Geometry check sheet. Reference: the model listing, model coordinates, mm. A direction names the side the tool comes from. Round coordinates to 2 decimals unless told otherwise and drop trailing zeros. Write each loop counter-clockwise with the first axis right and the second up, starting at its lowest first coordinate (ties: lowest second). Pieces come first, ordered by that corner, then holes. Notation, with made-up numbers: M 8.25,45 L 13.25,45 A30 ccw 13.25,77 Z; hole C -31.5,28.5 d5. An arc over 180 degrees is marked long. Answer in a Markdown table with one row per item. Add a question column.
from build123d import *

# Parameters (mm, degrees)
F0_W     = 96.5
F0_H     = 77
F1_DEPTH = 1.6
F2_W     = 81
F2_H     = 67
F3_DEPTH = 3.3
F4_W     = 45
F4_H     = 49
F5_DEPTH = 6.5


with BuildPart() as f1:
    # F0 (on Right) → F1 (new body, symmetric)
    with BuildSketch(Plane.YZ):
        Rectangle(F0_W, F0_H)
    extrude(amount=F1_DEPTH, both=True)

    # F2 (on face) → F3 (join)
    with BuildSketch(Plane.YZ.offset(1.6)):
        with Locations((-4.75, -5)):
            Rectangle(F2_W, F2_H)
    extrude(amount=F3_DEPTH)

    # F4 (on face) → F5 (join)
    with BuildSketch(Plane.YZ.offset(4.9)):
        with Locations((-22.75, -14)):
            Rectangle(F4_W, F4_H)
    extrude(amount=F5_DEPTH)


solid = f1.part
Item 1: Section check A-A, the plane z = 27. Record the boundary of the cut face in (x, y).
Item 2: Gauge pin test, flat ends, axial feed: pin 1 Ø1.6 at (x, y) = (4, -25) entering from +Z; pin 2 Ø5 at (x, y) = (9, -28.5) entering from +Z; pin 3 Ø1 at (x, z) = (8.5, 3) entering from +Y. Record the tip position at first contact, or that the pin passes through.
Item 3: Access from +Z, -Z, +X, -X, +Y, -Y to the whole of each face (thin tool, end or side, straight path). Record for faces 1 (the flat face through (0, 48.25, -1)), 2 (the flat face through (6, -45.25, -13)), 3 (the flat face through (3, 35.75, -5)), 4 (the flat face through (3, -5, 28.5)), 5 (the flat face through (0, -48.25, -1)).
Item 4: Scan lines: probe 1 along Z at (x, y) = (3.5, 30.5); probe 2 along Y at (x, z) = (10.25, 8); probe 3 along X at (y, z) = (-21, 17). Record each from-to range of solid material in increasing order. Write a range as from..to.
Item 5: Section check C-C, the plane x = 9.5. Record the boundary of the cut face in (y, z), and give its area (4 significant figures).
Item 6: Section check B-B, the plane y = -15. Record the boundary of the cut face in (x, z), and give its area (3 significant figures).
Item 7: Section check D-D, the plane y = 30. Record the boundary of the cut face in (x, z).
Result sheet:
| question | item | result |
|---|---|---|
| 1 | outline | M -1.6,-48.25 L 1.6,-48.25 L 1.6,-45.25 L 4.9,-45.25 L 4.9,35.75 L 1.6,35.75 L 1.6,48.25 L -1.6,48.25 Z |
| 2 | pin 1 | stops at z = 28.5 |
| 2 | pin 2 | stops at z = 10.5 |
| 2 | pin 3 | stops at y = -0.25 |
| 3 | face 1 | +Z, -Z, +X, -X, +Y |
| 3 | face 2 | +Z, -Z, +X, -Y |
| 3 | face 3 | +Z, -Z, +X, +Y |
| 3 | face 4 | +Z, +X, +Y, -Y |
| 3 | face 5 | +Z, -Z, +X, -X, -Y |
| 4 | probe 1 | z = -38.5..28.5 |
| 4 | probe 2 | y = -45.25..-0.25 |
| 4 | probe 3 | x = -1.6..4.9 |
| 5 | outline | M -45.25,-38.5 L -0.25,-38.5 L -0.25,10.5 L -45.25,10.5 Z |
| 5 | area | 2,205 mm^2 |
| 6 | outline | M -1.6,-38.5 L 11.4,-38.5 L 11.4,10.5 L 4.9,10.5 L 4.9,28.5 L 1.6,28.5 L 1.6,38.5 L -1.6,38.5 Z |
| 6 | area | 786 mm^2 |
| 7 | outline | M -1.6,-38.5 L 4.9,-38.5 L 4.9,28.5 L 1.6,28.5 L 1.6,38.5 L -1.6,38.5 Z |
